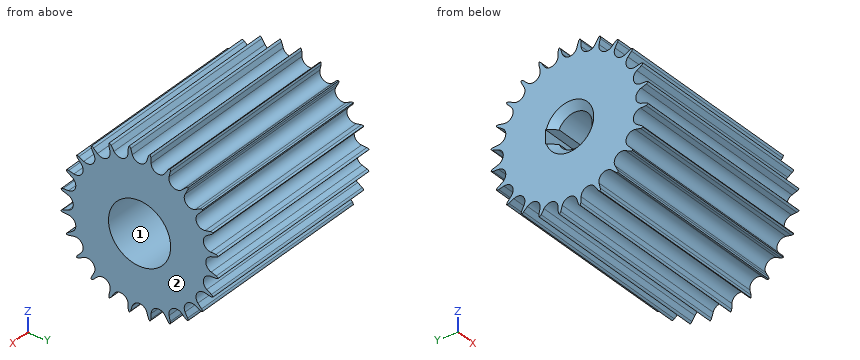
```python
from build123d import *

# Parameters (mm, degrees)
CHAMFER_1_SIZE           = 1
SKETCH_4_W               = 2
SKETCH_4_H               = 1.208712153
CUT_EXTRUDE_1_DEPTH      = 33.451810427
CUT_EXTRUDE_2_REACH      = 34.452
PATTERN_CIRCULAR_3_COUNT = 24


with BuildPart() as part:
    # Sketch 1 → Revolve 1 (revolve)
    with BuildSketch(Plane.XY, mode=Mode.PRIVATE) as revolve_1_sk:
        Polygon((0, 2.5), (0, 11.6), (28, 11.6), (28, 4.5), (20, 4.5), (20, 2.5), align=None)
    revolve(revolve_1_sk.sketch.rotate(Axis((0, 0, 0), (1, 0, 0)), 90), axis=Axis((0, 0, 0), (1, 0, 0)))

    # Chamfer 1
    chamfer_1_edges = [part.edges().sort_by_distance(p)[0] for p in [
        (0, 0, -2.5),
        (20, 0, -2.5),
    ]]
    chamfer(chamfer_1_edges, length=CHAMFER_1_SIZE)

    # Sketch 4 → Cut-Extrude 1 (cut, through all)
    with BuildSketch(Plane.ZY):
        with Locations((0, 2.895643923)):
            Rectangle(SKETCH_4_W, SKETCH_4_H)
    extrude(amount=-CUT_EXTRUDE_1_DEPTH, mode=Mode.SUBTRACT)

    # Sketch 6 → Cut-Extrude 2 (cut, up to next)
    with BuildSketch(Plane(origin=(0, 0, 0), x_dir=(0, 0, -1), z_dir=(1, 0, 0)), mode=Mode.PRIVATE) as cut_extrude_2_sk1:
        with BuildLine():
            Line((1.282657956, 11.110010829), (1.049088646, 10.369223621))
            ThreePointArc((1.049088646, 10.369223621), (0, 9.6), (-1.049088646, 10.369223621))
            Line((-1.049088646, 10.369223621), (-1.282657956, 11.110010829))
            ThreePointArc((-1.282657956, 11.110010829), (-1.496857499, 11.385110965), (-1.838773928, 11.453336215))
            ThreePointArc((-1.838773928, 11.453336215), (-2.085185987, 11.411047253), (-2.330629413, 11.363457508))
            Line((-2.330629413, 11.363457508), (-2.815847343, 12.902372174))
            ThreePointArc((-2.815847343, 12.902372174), (0, 13.206066938), (2.815847343, 12.902372174))
            Line((2.815847343, 12.902372174), (2.330629413, 11.363457508))
            ThreePointArc((2.330629413, 11.363457508), (2.085185987, 11.411047253), (1.838773928, 11.453336215))
            ThreePointArc((1.838773928, 11.453336215), (1.496857499, 11.385110965), (1.282657956, 11.110010829))
        make_face()
    cut_extrude_2_tool1 = extrude(cut_extrude_2_sk1.sketch, amount=CUT_EXTRUDE_2_REACH, mode=Mode.PRIVATE) & part.part
    cut_extrude_2 = cut_extrude_2_tool1.solids().sort_by_distance((0, 11.799996, 0))[0]
    add(cut_extrude_2, mode=Mode.SUBTRACT)

    # Pattern Circular 3: Cut-Extrude 2 ×24 about axis
    pattern_circular_3_axis = Axis((0, 0, 0), (1, 0, 0))
    for i in range(1, PATTERN_CIRCULAR_3_COUNT):
        add(cut_extrude_2.rotate(pattern_circular_3_axis, i * 360 / PATTERN_CIRCULAR_3_COUNT), mode=Mode.SUBTRACT)


solid = part.part
```
CAD build for the part. Positions are in the model's coordinates, mm. Face numbers are marked on the shaded views. Round coordinates to 2 decimals unless told otherwise and drop trailing zeros. Order: outer loops, then holes, each group sorted by start corner. A loop starts at its lowest first (then second) coordinate and runs counter-clockwise, first axis right, second up.
Item 1: Saw through at A-A on y = 0. Write the cut outline in (x, z), then the cut area to 3 significant figures.
Item 2: Saw through at B-B on z = 0. Write the cut outline in (x, y), then the cut area to 3 significant figures.
Item 3: Mould opens along Y. For the marked faces 1 and 2 say: pulls with the +Y half, pulls with the -Y half, needs draft (parallel to the pull), parting line crosses it, or undercut.
Item 4: Pin check, flat tips, straight feed: pin 1 (5 mm diameter, centred on x = 18.5, z = 6, fed in from -Y); pin 2 (5 mm diameter, centred on x = 25, z = 5, fed in from +Y); pin 3 (1.5 mm diameter, centred on x = 16.5, y = -8.5, fed in from -Z). Stop position of each tip, or through.
Item 5: Saw through at C-C on z = -5.75. Write the cut outline in (x, y), then the cut area to 3 significant figures.
Item 6: Probe line 1 along Z through (x, y) = (9.5, 0); line 2 along Z through (x, y) = (21, 9.5); line 3 along Y through (x, z) = (21.5, 10). List the from-to ranges inside material, lowest first.
Reported:
1. outline: (0, -9.6) - (28, -9.6) - (28, -4.5) - (20, -4.5) - (20, -3.5) - (19, -2.5) - (1, -2.5) - (0, -3.5) - close; (0, 3.5) - (1, 2.5) - (19, 2.5) - (20, 3.5) - (20, 4.5) - (28, 4.5) - (28, 9.6) - (0, 9.6) - close
1. area: 364 mm2
2. outline: (0, -9.6) - (28, -9.6) - (28, -4.5) - (20, -4.5) - (20, -3.5) - (19, -2.5) - (1, -2.5) - (0, -3.5) - close; (0, 3.5) - (20, 3.5) - (20, 4.5) - (28, 4.5) - (28, 9.6) - (0, 9.6) - close
2. area: 345 mm2
3. face 1: undercut
3. face 2: needs draft
4. pin 1: stops at y = -10.61
4. pin 2: stops at y = 10.61
4. pin 3: stops at z = -7.01
5. outline: (0, -8.24) - (28, -8.24) - (28, 8.24) - (0, 8.24) - close
5. area: 462 mm2
6. line 1: z = -9.6 to -2.5, 2.5 to 9.6
6. line 2: z = -4.28 to -3.48, -2.05 to 2.05, 3.48 to 4.28
6. line 3: y = -4.39 to -3.86, -1.72 to -0.85, 0.85 to 1.72, 3.86 to 4.39
